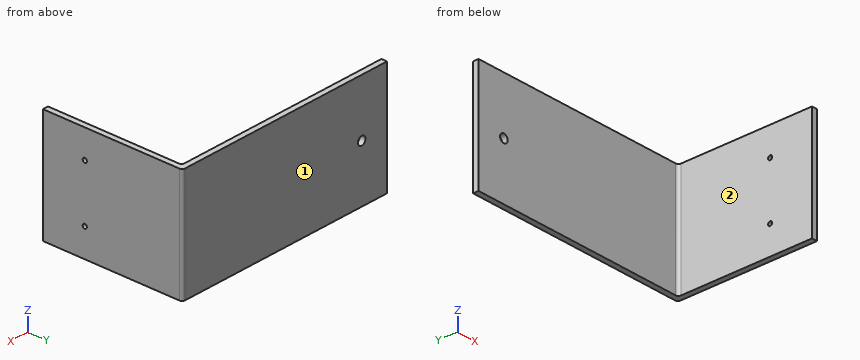
from build123d import *

# Parameters (mm, degrees)
SKETCH1_W           = 80
SKETCH1_H           = 40
SKETCH1_R           = 1.5
BOSS_EXTRUDE1_DEPTH = 2
SKETCH2_W           = 1
SKETCH2_H           = 40
BOSS_EXTRUDE2_DEPTH = 50
SKETCH3_R           = 0.75
CUT_EXTRUDE1_DEPTH  = 70
FILLET1_R           = 1


with BuildPart() as part:
    # Sketch1 → Boss-Extrude1 (new body)
    with BuildSketch(Plane(origin=(0, 0, 0), x_dir=(1, 0, 0), z_dir=(0, 1, 0))):
        with Locations((40, 20)):
            Rectangle(SKETCH1_W, SKETCH1_H)
        with Locations(Location((10, 20, 0), (0, 0, 270))):
            Circle(SKETCH1_R, mode=Mode.SUBTRACT)
    extrude(amount=BOSS_EXTRUDE1_DEPTH)

    # Sketch2 → Boss-Extrude2 (add)
    with BuildSketch(Plane(origin=(0, 2, 0), x_dir=(1, 0, 0), z_dir=(0, 1, 0))):
        with Locations((79.5, 20)):
            Rectangle(SKETCH2_W, SKETCH2_H)
        with Locations((80.5, 20)):
            Rectangle(SKETCH2_W, SKETCH2_H)
    extrude(amount=-BOSS_EXTRUDE2_DEPTH)

    # Sketch3 → Cut-Extrude1 (cut)
    with BuildSketch(Plane.ZY.offset(-79)):
        with Locations((-30, -33)):
            Circle(SKETCH3_R)
        with Locations((-10, -33)):
            Circle(SKETCH3_R)
    extrude(amount=-CUT_EXTRUDE1_DEPTH, mode=Mode.SUBTRACT)

    # Fillet1
    fillet1_edges = [part.edges().sort_by_distance(p)[0] for p in [
        (79, 0, -20),
        (81, 2, -20),
    ]]
    fillet(fillet1_edges, radius=FILLET1_R)


solid = part.part
Check sheet for the modelled part. Datum: model origin and axes. Units: mm. Face numbers are marked on the shaded views. A direction names the side the tool comes from. Give positions to 0.01 mm unless a question says otherwise; leave off trailing zeros. Loops run counter-clockwise (first coordinate to the right, second up) from the corner with the lowest first, then second, coordinate; pieces in that order, holes last. Notation, with made-up numbers: M -6.75,-38.75 L -0.75,-38.75 A29 ccw -0.75,-3.75 Z; hole C 7,-3.75 d11. An arc over 180 degrees is marked long. Use a Markdown table: item, result. Add a question column.
Q1. Sectioned sample at C-C, the plane x = 42.5. Record the cut outline in (y, z), then the cut area to 3 significant figures.
Q2. Scan lines: line 1 along Z through (x, y) = (80.55, -33); line 2 along Y through (x, z) = (80, -30); line 3 along Y through (x, z) = (66.5, -29.5). Record each from-to range of solid material in increasing order. Write a range as [from, to].
Q3. Sectioned sample at A-A, the plane z = -20. Record the cut outline in (x, y), then the cut area to 3 significant figures.
Q4. Go/stop test with flat-tipped pins: pin 1 (8 mm diameter, centred on x = 21, y = -5.5, fed in from -Z); pin 2 (3 mm diameter, centred on x = 34, z = -29.5, fed in from -Y). Record where each tip stops, or that it passes through.
Q5. Sectioned sample at D-D, the plane y = -45. Record the cut outline in (x, z), then the cut area to 3 significant figures.
Q6. Tool access check on the marked faces 1 and 2. Record the directions out of +Z, -Z, +X, -X, +Y, -Y that give a thin tool (end or side, any length) a straight path to the whole face; none if there is none.
Q7. Sectioned sample at B-B, the plane z = -36.5. Record the cut outline in (x, y).
Verdict:
| question | item | result |
|---|---|---|
| 1 | outline | M 0,-40 L 2,-40 L 2,0 L 0,0 Z |
| 1 | area | 80.0 mm^2 |
| 2 | line 1 | [-40, -30.75], [-29.25, -10.75], [-9.25, 0] |
| 2 | line 2 | [-48, -33.75], [-32.25, 2] |
| 2 | line 3 | [0, 2] |
| 3 | outline | M 0,0 L 8.5,0 L 8.5,2 L 0,2 Z; M 11.5,0 L 78,0 A1 cw 79,-1 L 79,-48 L 81,-48 L 81,1 A1 ccw 80,2 L 11.5,2 Z |
| 3 | area | 252 mm^2 |
| 4 | pin 1 | through |
| 4 | pin 2 | y = 0 |
| 5 | outline | M 79,-40 L 81,-40 L 81,0 L 79,0 Z |
| 5 | area | 80.0 mm^2 |
| 6 | face 1 | +Z, -Z, +X, -X, +Y |
| 6 | face 2 | +Z, -Z, -X, -Y |
| 7 | outline | M 0,0 L 78,0 A1 cw 79,-1 L 79,-48 L 81,-48 L 81,1 A1 ccw 80,2 L 0,2 Z |
